Verification items for the finished model (mm, model axes). Coordinates: 2 decimals unless noted, no trailing zeros. Write each loop counter-clockwise with the first axis right and the second up, starting at its lowest first coordinate (ties: lowest second). Pieces come first, ordered by that corner, then holes. Notation, with made-up numbers: (-26.75, 30) - (20.25, 30) arc R6 cw to (20.25, 37) - close; hole circle Ø9 at (-29.5, 57). An arc over 180 degrees is marked (long way). Use one line per item in the form item = value. Start each with the question number.
(1) Sectioned sample at C-C (y = 2). Count the separate pieces of the cut face and the enclosed holes in it, and give its area (3 significant figures).
(2) Sectioned sample at A-A (x = 15). Record the cut outline in (y, z) (3 decimals), and give its area (3 significant figures).
(3) Sectioned sample at B-B (z = -110.5). Record the cut outline in (x, y) (3 decimals), and give its area (3 significant figures).
(4) Material ranges on line 1 (Z direction, x = 76.2, y = 2.35); line 2 (Z direction, x = 89, y = 1.4); line 3 (X direction, y = 0.4, z = -63), recorded low to high. Write a range as [from, to].
from build123d import *

# Parameters (mm, degrees)
SKETCH1_W           = 152.4
SKETCH1_H           = 152.4
SKETCH1_R           = 1.6637
BOSS_EXTRUDE4_DEPTH = 3.175


with BuildPart() as part:
    # Sketch1 → Boss-Extrude4 (new body)
    with BuildSketch(Plane(origin=(0, 0, 0), x_dir=(1, 0, 0), z_dir=(0, 1, 0))):
        with Locations((76.2, 76.2)):
            Rectangle(SKETCH1_W, SKETCH1_H)
        with Locations(Location((7.62, 7.62, 0), (0, 0, 270))):
            Circle(SKETCH1_R, mode=Mode.SUBTRACT)
        with Locations(Location((7.62, 144.78, 0), (0, 0, 270))):
            Circle(SKETCH1_R, mode=Mode.SUBTRACT)
        with Locations(Location((144.78, 144.78, 0), (0, 0, 270))):
            Circle(SKETCH1_R, mode=Mode.SUBTRACT)
        with Locations(Location((144.78, 7.62, 0), (0, 0, 270))):
            Circle(SKETCH1_R, mode=Mode.SUBTRACT)
        with Locations(Location((76.2, 7.62, 0), (0, 0, 270))):
            Circle(SKETCH1_R, mode=Mode.SUBTRACT)
        with Locations(Location((76.2, 144.78, 0), (0, 0, 270))):
            Circle(SKETCH1_R, mode=Mode.SUBTRACT)
        with Locations(Location((144.78, 76.2, 0), (0, 0, 270))):
            Circle(SKETCH1_R, mode=Mode.SUBTRACT)
        with Locations(Location((7.62, 76.2, 0), (0, 0, 270))):
            Circle(SKETCH1_R, mode=Mode.SUBTRACT)
        Polygon((69.85, 7.62), (20.32, 7.62), (7.62, 20.32), (7.62, 69.85), (13.119261314, 73.025), (13.119261314, 79.375), (7.62, 82.55), (7.62, 132.08), (20.32, 144.78), (69.85, 144.78), (73.025, 139.280738686), (79.375, 139.280738686), (82.55, 144.78), (132.08, 144.78), (144.78, 132.08), (144.78, 82.55), (139.280738686, 79.375), (139.280738686, 73.025), (144.78, 69.85), (144.78, 20.32), (132.08, 7.62), (82.55, 7.62), (79.375, 13.119261314), (73.025, 13.119261314), align=None, mode=Mode.SUBTRACT)
    extrude(amount=BOSS_EXTRUDE4_DEPTH)


solid = part.part
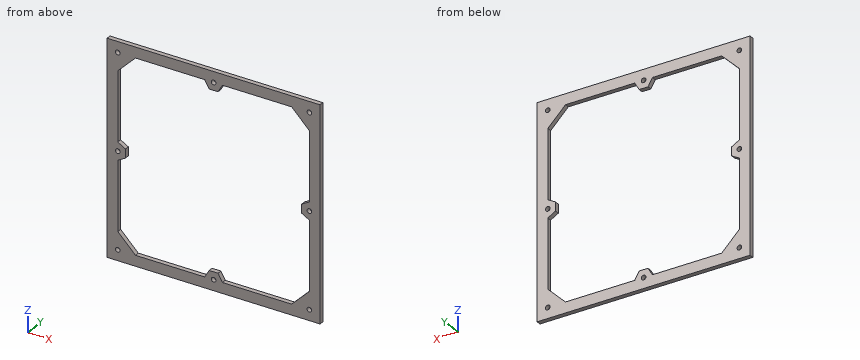
Answers below:
q1.separate_pieces = 1
q1.enclosed_holes = 9
q1.area = 4,880 mm2
q2.outline = (0, -152.4) - (3.175, -152.4) - (3.175, -139.46) - (0, -139.46) - close; (0, -12.94) - (3.175, -12.94) - (3.175, 0) - (0, 0) - close
q2.area = 82.2 mm2
q3.outline = (0, 0) - (7.62, 0) - (7.62, 3.175) - (0, 3.175) - close; (144.78, 0) - (152.4, 0) - (152.4, 3.175) - (144.78, 3.175) - close
q3.area = 48.4 mm2
q4.line_1 = [-152.4, -146.44], [-143.12, -139.28], [-13.12, -9.28], [-5.96, 0]
q4.line_2 = [-152.4, -144.78], [-7.62, 0]
q4.line_3 = [0, 7.62], [144.78, 152.4]
